Could you check a few things on this model? Use its own coordinates, in mm. A direction names the side the tool comes from. Round coordinates to 2 decimals unless told otherwise and drop trailing zeros. Write each loop counter-clockwise with the first axis right and the second up, starting at its lowest first coordinate (ties: lowest second). Pieces come first, ordered by that corner, then holes. Notation, with made-up numbers: (13, 70.5) - (27, 70.5) arc R22 ccw to (27, 89.5) - close; hole circle Ø9 at (82.25, 66.5). An arc over 180 degrees is marked (long way). Write each question's results on one line, items separated by ' | '. Start each with the question number.
(1) Imagine slicing it at C-C on y = 9. Write out the boundary of the cut face in (x, z).
(2) Imagine slicing it at A-A on x = 6.5. Write out the boundary of the cut face in (y, z).
(3) Imagine slicing it at B-B on z = 1.25. Write out the boundary of the cut face in (x, y), then the cut area to 3 significant figures.
(4) For P1, Ø3.5, axis at x = 7, y = 9.5, coming from the +Z side; P2, Ø6, axis at x = 7, y = 6.5, coming from the -Z side, each with a flat end and sliding along its axis, tell me the tip position at first contact or that it passes through.
(5) Imagine slicing it at D-D on x = 4.01. Write out the boundary of the cut face in (y, z).
(6) Thinking about a two-plate mould opening in Y: for faces 4 (the flat face through (13, 6, 1.9)), 5 (the flat face through (6, 0.15, 1)), 6 (the cylindrical face through (3.61, 12.42, -0.1)), which applies, +Y half, -Y half, draft (parallel to the pull), parting line (faces both ways), or undercut?
(7) Please list where these lines run through material, in increasing order: line 1 (Y direction, x = 5, z = 1.6); line 2 (Y direction, x = 4.75, z = 1.85); line 3 (X direction, y = 12.25, z = 1.25). Write a range as [from, to].
(8) On a 3-axis mill with a long thin cutter (end or side, diameter ignored), from which of +Z, -Z, +X, -X, +Y, -Y can I reach the whole of each face in a straight line? I mean faces 1 (the flat face through (14, 0.95, 1)), 2 (the flat face through (0.71, 10.4, 0.6)), 3 (the flat face through (6.6, 13.9, 1.4)). Say none if no direction works.
```python
from build123d import *

# Parameters (mm, degrees)
PAD_DEPTH       = 1.85
SKETCH_W        = 4.4
SKETCH_H        = 1.85
POCKET001_DEPTH = 0.4
SKETCH005_W     = 11.2
SKETCH005_H     = 0.9
POCKET002_DEPTH = 12.6
SKETCH006_R     = 0.4
PAD003_DEPTH    = 0.4
SKETCH008_W     = 0.2
SKETCH008_H     = 0.4
POCKET003_DEPTH = 0.3
CHAMFER_SIZE    = 0.1
CHAMFER001_SIZE = 0.2


with BuildPart() as part:
    # Sketch004 → Pad (new body)
    with BuildSketch(Plane.XY.offset(0.05)):
        with BuildLine():
            Line((0.71, 14.65), (0.71, 5.95))
            ThreePointArc((0.634493, 5.41274), (0.691031, 5.67873), (0.71, 5.95))
            Line((0.634493, 5.41274), (0, 3.2))
            Line((0, 3.2), (0, 0.15))
            Line((0, 0.15), (13, 0.15))
            Line((13, 0.15), (13, 0.95))
            Line((13, 0.95), (14.5, 0.95))
            Line((14.5, 0.95), (14.5, 14.65))
            Line((0.71, 14.65), (14.5, 14.65))
        make_face()
    extrude(amount=PAD_DEPTH)

    # Sketch (on Face11 of Pad) → Pocket001 (cut)
    with BuildSketch(Plane.XY.offset(1.95)):
        with Locations((3.9, 1.425)):
            Rectangle(SKETCH_W, SKETCH_H)
    extrude(amount=-POCKET001_DEPTH, mode=Mode.SUBTRACT)

    # Sketch005 (on Face8 of Pocket001) → Pocket002 (cut)
    with BuildSketch(Plane(origin=(-0.05, 0, 0), x_dir=(0, -1, 0), z_dir=(-1, 0, 0))):
        with Locations((-8.3, 1.45)):
            Rectangle(SKETCH005_W, SKETCH005_H)
    extrude(amount=-POCKET002_DEPTH, mode=Mode.SUBTRACT)

    # Sketch006 → Pad003 (join)
    with BuildSketch(Plane.XY.offset(0.05)):
        with Locations((4.01, 4.4)):
            Circle(SKETCH006_R)
        with Locations((4.01, 12.4)):
            Circle(SKETCH006_R)
    extrude(amount=-PAD003_DEPTH)

    # Sketch008 → Pocket003 (cut)
    with BuildSketch(Plane.XY.offset(0.05)):
        with Locations((14.4, 5.2)):
            Rectangle(SKETCH008_W, SKETCH008_H)
        with Locations((14.4, 6.3)):
            Rectangle(SKETCH008_W, SKETCH008_H)
        with Locations((14.4, 7.4)):
            Rectangle(SKETCH008_W, SKETCH008_H)
        with Locations((14.4, 8.5)):
            Rectangle(SKETCH008_W, SKETCH008_H)
        with Locations((14.4, 9.6)):
            Rectangle(SKETCH008_W, SKETCH008_H)
        with Locations((14.4, 10.7)):
            Rectangle(SKETCH008_W, SKETCH008_H)
        with Locations((14.4, 11.8)):
            Rectangle(SKETCH008_W, SKETCH008_H)
        with Locations((14.4, 12.9)):
            Rectangle(SKETCH008_W, SKETCH008_H)
        with Locations((14.4, 14)):
            Rectangle(SKETCH008_W, SKETCH008_H)
    extrude(amount=POCKET003_DEPTH, mode=Mode.SUBTRACT)

    # Chamfer
    chamfer_edges = [part.edges().sort_by_distance(p)[0] for p in [
        (3.61, 12.4, -0.35),
        (3.61, 4.4, -0.35),
    ]]
    chamfer(chamfer_edges, length=CHAMFER_SIZE)

    # Chamfer001
    chamfer001_edges = [part.edges().sort_by_distance(p)[0] for p in [
        (7.605, 14.65, 1.9),
        (14.5, 7.8, 1.9),
        (13.75, 0.95, 1.9),
        (13, 0.55, 1.9),
        (6.5, 0.15, 1.9),
        (0.71, 13.9, 1.45),
        (0.71, 9.925, 1),
        (0.691031, 5.67873, 1),
        (0.317247, 4.30637, 1),
        (0, 2.95, 1),
        (0, 2.7, 1.45),
    ]]
    chamfer(chamfer001_edges, length=CHAMFER001_SIZE)


solid = part.part
```
Response:
1) outline: (0.71, 0.05) - (14.5, 0.05) - (14.5, 1.7) - (14.3, 1.9) - (12.55, 1.9) - (12.55, 1) - (0.91, 1) - (0.71, 0.8) - close
2) outline: (0.15, 0.05) - (14.65, 0.05) - (14.65, 1.7) - (14.45, 1.9) - (13.9, 1.9) - (13.9, 1) - (2.7, 1) - (2.7, 1.9) - (0.35, 1.9) - (0.15, 1.7) - close
3) outline: (0, 0.15) - (13, 0.15) - (13, 0.95) - (14.5, 0.95) - (14.5, 14.65) - (0.71, 14.65) - (0.71, 14.1) - (0.91, 13.9) - (12.55, 13.9) - (12.55, 2.7) - (0.2, 2.7) - (0, 2.5) - close | area: 67.9 mm²
4) P1: z = 1 | P2: z = 0.05
5) outline: (0.15, 0.05) - (4, 0.05) - (4, -0.25) - (4.1, -0.35) - (4.7, -0.35) - (4.8, -0.25) - (4.8, 0.05) - (12, 0.05) - (12, -0.25) - (12.1, -0.35) - (12.7, -0.35) - (12.8, -0.25) - (12.8, 0.05) - (14.65, 0.05) - (14.65, 1.7) - (14.45, 1.9) - (13.9, 1.9) - (13.9, 1) - (2.7, 1) - (2.7, 1.9) - (2.35, 1.9) - (2.35, 1.55) - (0.5, 1.55) - (0.5, 1.9) - (0.35, 1.9) - (0.15, 1.7) - close
6) face 4: draft | face 5: -Y half | face 6: undercut
7) line 1: [0.15, 0.5], [2.35, 2.7], [13.9, 14.65] | line 2: [0.3, 0.5], [2.35, 2.7], [13.9, 14.5] | line 3: [12.55, 14.5]
8) face 1: +Z, -Z, +X, -Y | face 2: +Z, -Z, -X, +Y | face 3: +Z, -X
